from build123d import *

# Parameters (mm, degrees)
SKETCH_R      = 30
PAD_DEPTH     = 10
SKETCH001_R   = 3.4
HOLE_DEPTH    = 10.001
SKETCH002_R   = 1.25
HOLE001_DEPTH = 10.001


with BuildPart() as part:
    # Sketch → Pad (new body)
    with BuildSketch(Plane.XY):
        Circle(SKETCH_R)
    extrude(amount=PAD_DEPTH)

    # Sketch001 → Hole (cut, through all)
    with BuildSketch(Plane.XY):
        Circle(SKETCH001_R)
    extrude(amount=HOLE_DEPTH, mode=Mode.SUBTRACT)

    # Sketch002 → Hole001 (cut, through all)
    with BuildSketch(Plane.XY):
        with Locations((-14.295, 10)):
            Circle(SKETCH002_R)
        with Locations((14.295, 10)):
            Circle(SKETCH002_R)
        with Locations((14.295, -10)):
            Circle(SKETCH002_R)
        with Locations((-14.295, -10)):
            Circle(SKETCH002_R)
    extrude(amount=HOLE001_DEPTH, mode=Mode.SUBTRACT)


solid = part.part
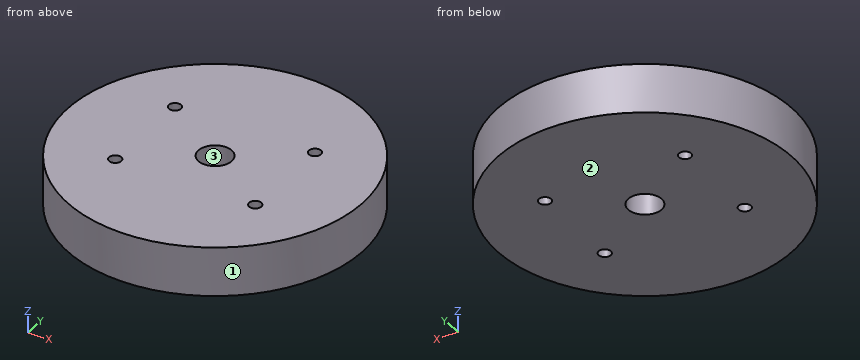
Design review of the part built by this model. Coordinates are the model's own, in mm. Face numbers are marked on the shaded views. Round coordinates to 2 decimals unless told otherwise and drop trailing zeros. Loops run counter-clockwise (first coordinate to the right, second up) from the corner with the lowest first, then second, coordinate; pieces in that order, holes last. Notation, with made-up numbers: (63, 51.5) - (74, 51.5) arc R33 cw to (74, 89.5) - close; hole circle Ø11 at (4, 41). An arc over 180 degrees is marked (long way). One line per item, written item: value. Start each with the question number.
1) Insertion check: pin 1 Ø4 at (y, z) = (-14, 6.5) entering from -X; pin 2 Ø4 at (x, y) = (14.295, -10) entering from -Z; pin 3 Ø2 at (x, y) = (-14.295, -10) entering from +Z; pin 4 Ø6 at (y, z) = (-7, 6) entering from +X. Each pin has a flat end and moves straight along its axis. Give the tip position at first contact, or say it passes through.
2) Draft analysis for pull direction Y (two halves, no side actions). For the marked faces 1, 2 and 3, state which applies: +Y half, -Y half, draft (parallel to the pull), parting line (faces both ways), or undercut.
3) Consider section B-B on z = 1.25. Give the boundary of the cut face in (x, y) (3 decimals).
4) Consider section D-D on x = -16.5. Give the boundary of the cut face in (y, z), then the cut area to 3 significant figures.
5) To check wall thickness, follow L1, parallel to X at y = 10, z = 5.75 (3 decimals); L2, parallel to Y at x = 0, z = 2.75; L3, parallel to X at y = 1, z = 0.75. State the ranges of each line that lie inside material, in increasing order. Write a range as from..to.
6) Consider section C-C on y = 10. Give the boundary of the cut face in (x, z) (3 decimals), then the cut area to 3 significant figures.
7) Consider section A-A on y = 0. Give the boundary of the cut face in (x, z), then the cut area to 3 significant figures.
Reported:
1. pin 1: stops at x = -27.5
1. pin 2: stops at z = 0
1. pin 3: passes through
1. pin 4: stops at x = 29.73
2. face 1: parting line
2. face 2: draft
2. face 3: undercut
3. outline: circle Ø60 at (0, 0); hole circle Ø2.5 at (-14.295, -10); hole circle Ø2.5 at (-14.295, 10); hole circle Ø6.8 at (0, 0); hole circle Ø2.5 at (14.295, -10); hole circle Ø2.5 at (14.295, 10)
4. outline: (-25.05, 0) - (25.05, 0) - (25.05, 10) - (-25.05, 10) - close
4. area: 501 mm^2
5. L1: x = -28.284..-15.545, -13.045..13.045, 15.545..28.284
5. L2: y = -30..-3.4, 3.4..30
5. L3: x = -29.98..-3.25, 3.25..29.98
6. outline: (-28.284, 0) - (-15.545, 0) - (-15.545, 10) - (-28.284, 10) - close; (-13.045, 0) - (13.045, 0) - (13.045, 10) - (-13.045, 10) - close; (15.545, 0) - (28.284, 0) - (28.284, 10) - (15.545, 10) - close
6. area: 516 mm^2
7. outline: (-30, 0) - (-3.4, 0) - (-3.4, 10) - (-30, 10) - close; (3.4, 0) - (30, 0) - (30, 10) - (3.4, 10) - close
7. area: 532 mm^2
